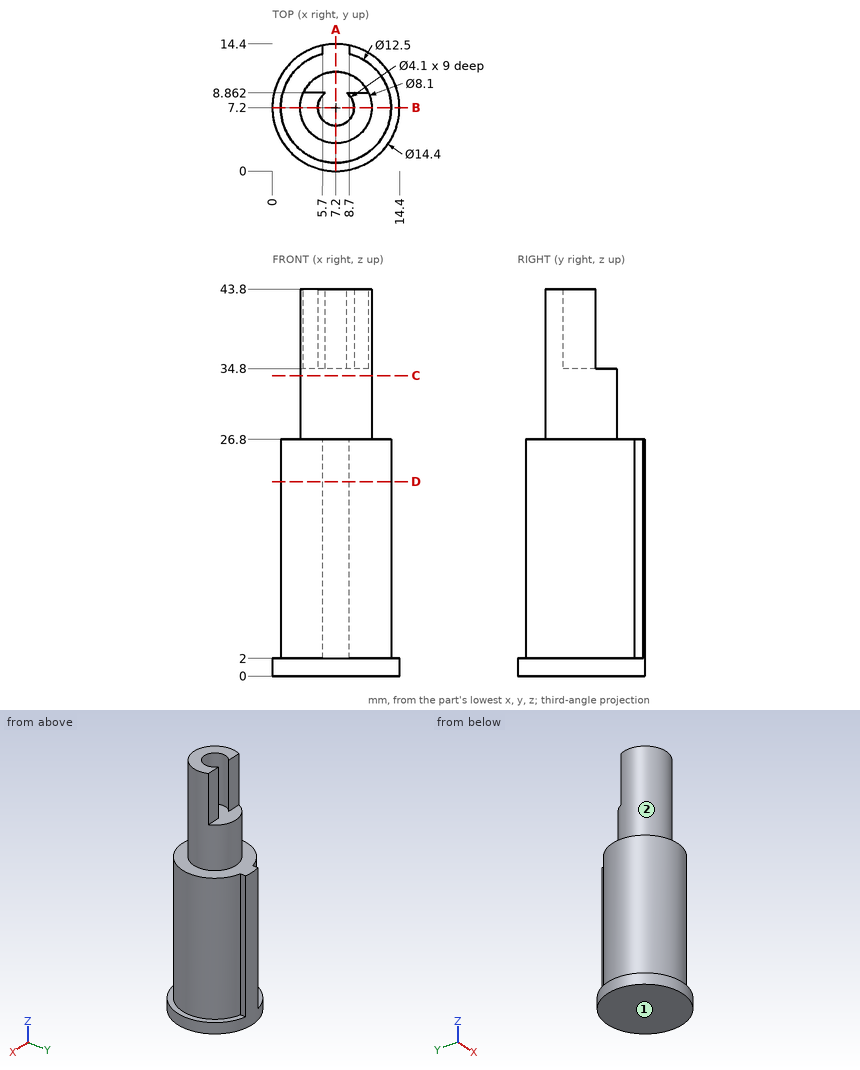
Design review of the part shown in the three views and the two pictorial views. Dimensions are in mm from the part's minimum x, y and z. A direction names the side the tool comes from. Coordinates: 2 decimals unless noted, no trailing zeros. Write each loop counter-clockwise with the first axis right and the second up, starting at its lowest first coordinate (ties: lowest second). Pieces come first, ordered by that corner, then holes.
1) Machinability: for the marked faces 1 and 2, which of the approach directions +Z, -Z, +X, -X, +Y, -Y give a long, thin tool a straight path to every point of the face, cutting with its end or side? Answer none if there is none.
2) We need section C-C on z = 34. State the section outline as (x, y) points, then the cut area to 3 significant figures.
3) We need section D-D on z = 22. State the section outline as (x, y) points, then the cut area to 3 significant figures.
4) We need section B-B on y = 7.2. State the section outline as (x, z) points.
5) Clearance check with flat-ended pins moving along their axes: pin 1 Ø6 at (y, z) = (11, 25) entering from +X; pin 2 Ø0.8 at (y, z) = (14, 10.5) entering from +X; pin 3 Ø4 at (x, z) = (8, 39) entering from +Y; pin 4 Ø6 at (x, y) = (8, 11) entering from +Z. State where each tip first meets the part, or that it passes through.
6) We need section A-A on x = 7.2. State the section outline as (y, z) points, then the cut area to 3 significant figures.
7) To check wall thickness, follow probe 1 along X at (y, z) = (7.2, 40.75); probe 2 along Z at (x, y) = (12, 3.5); probe 3 along X at (y, z) = (7, 30.5) (3 decimals). State the ranges of each line that lie inside material, in increasing order.
Answer list:
1. face 1: -Z, +X, -X, +Y, -Y
1. face 2: +Z
2. outline: circle Ø8.1 at (7.2, 7.2)
2. area: 51.5 mm2
3. outline: (5.7, 13.27) arc R6.25 ccw (long way) to (8.7, 13.27) - (8.7, 14.24) arc R7.2 ccw to (5.7, 14.24) - close
3. area: 126 mm2
4. outline: (0, 0) - (14.4, 0) - (14.4, 2) - (13.45, 2) - (13.45, 26.8) - (11.25, 26.8) - (11.25, 43.8) - (9.25, 43.8) - (9.25, 34.8) - (5.15, 34.8) - (5.15, 43.8) - (3.15, 43.8) - (3.15, 26.8) - (0.95, 26.8) - (0.95, 2) - (0, 2) - close
5. pin 1: stops at x = 13.4
5. pin 2: stops at x = 8.7
5. pin 3: stops at y = 8.86
5. pin 4: stops at z = 43.8
6. outline: (0, 0) - (14.4, 0) - (14.4, 26.8) - (11.25, 26.8) - (11.25, 34.8) - (5.15, 34.8) - (5.15, 43.8) - (3.15, 43.8) - (3.15, 26.8) - (0.95, 26.8) - (0.95, 2) - (0, 2) - close
6. area: 445 mm2
7. probe 1: x = 3.15 to 5.15, 9.25 to 11.25
7. probe 2: z = 0 to 26.8
7. probe 3: x = 3.155 to 11.245
